Read the model definition and answer for the solid it produces. Units are mm, in the model's axes. Face numbers are marked on the shaded views. A direction names the side the tool comes from. Give positions to 0.01 mm unless a question says otherwise; leave off trailing zeros. Write each loop counter-clockwise with the first axis right and the second up, starting at its lowest first coordinate (ties: lowest second). Pieces come first, ordered by that corner, then holes. Notation, with made-up numbers: (48.25, -14) - (77.25, -14) arc R25 ccw to (77.25, 14) - close; hole circle Ø9 at (88.5, 84). An arc over 180 degrees is marked (long way). Answer as a JSON object with one key per item and string values. Group by question number.
```python
from build123d import *

# Parameters (mm, degrees)
F1_DEPTH     = 25
F2_R         = 5
F3_R         = 5
F4_R         = 2
F6_R         = 5
F7_DEPTH     = 20
F8_T1_DEPTH  = 16.879655815
F8_T3_DEPTH  = 23.3726224193
F8_T5_DEPTH  = 33.0268060681
F8_T10_DEPTH = 5.1
F8_T16_DEPTH = 5.1
F8_T22_DEPTH = 98.4210661838
F8_S23_R     = 20
F8_T24_DEPTH = 53
F8_S25_R     = 20
F8_T26_DEPTH = 53
F8_T30_DEPTH = 70.867251183
F8_S31_R     = 20
F8_T32_DEPTH = 39
F8_S33_R     = 20
F8_T34_DEPTH = 39


# Not quite as in the source:
# - a fillet or chamfer that OpenCascade refuses, or shapes differently, is made with other operations: its cross-section is extruded or revolved along the edge and cut away or added
# - two fillets or chamfers of one size are made in one step


with BuildPart() as f1:
    # F0 (on Top) → F1 (new body)
    with BuildSketch(Plane.XY):
        with BuildLine():
            ThreePointArc((-62.7989065684, 39.6886658546), (-81.243248627, 20.090620438), (-63.3367104763, 0))
            Line((-63.3367104763, 0), (0, -156.2183324342))
            Line((0, -156.2183324342), (63.3367104763, 0))
            ThreePointArc((63.3367104763, 0), (83.9060549488, 20.1553189736), (63.1791622356, 40.1485861756))
            ThreePointArc((63.1791622356, 40.1485861756), (68.8985621757, 62.3156526678), (50.0641206725, 75.3292680691))
            ThreePointArc((50.0641206725, 75.3292680691), (54.0847867027, 97.4676528526), (34.9687938538, 109.335788913))
            ThreePointArc((34.9687938538, 109.335788913), (37.8165399559, 130.8078112166), (19.4443891765, 142.2804515145))
            ThreePointArc((19.4443891765, 142.2804515145), (6.5496116272, 157.6455026462), (10.1508991793, 177.3784905672))
            ThreePointArc((10.1508991793, 177.3784905672), (-12.7726518652, 165.7418593556), (-21.8806297798, 141.7013702435))
            ThreePointArc((-21.8806297798, 141.7013702435), (-36.0248561638, 134.2091888045), (-40.144512278, 118.7424387834))
            Line((-40.144512278, 118.7424387834), (-34.6308081302, 107.732548238))
            ThreePointArc((-34.6308081302, 107.732548238), (-50.0933619749, 100.6048777691), (-54.4620472952, 84.1486070408))
            Line((-54.4620472952, 84.1486070408), (-50.2881059675, 75.0966394345))
            ThreePointArc((-50.2881059675, 75.0966394345), (-68.9068668709, 61.7610342158), (-62.7989065684, 39.6886658546))
        make_face()
        with BuildLine():
            Line((-19.4251702535, 141.7357782283), (-21.8806297798, 141.7013702435))
            ThreePointArc((-21.8806297798, 141.7013702435), (-20.6534286134, 141.7562965225), (-19.4251702535, 141.7357782283))
        make_face(mode=Mode.SUBTRACT)
        with BuildLine():
            ThreePointArc((-40.144512278, 118.7424387834), (-38.2560486822, 112.8026084286), (-34.6308081302, 107.732548238))
            Line((-34.6308081302, 107.732548238), (-40.144512278, 118.7424387834))
        make_face()
        with BuildLine():
            ThreePointArc((-54.4620472952, 84.1486070408), (-52.9480489841, 79.3584206811), (-50.2881059675, 75.0966394345))
            Line((-50.2881059675, 75.0966394345), (-54.4620472952, 84.1486070408))
        make_face()
        with BuildLine():
            ThreePointArc((-19.4251702535, 141.7357782283), (-20.6534286134, 141.7562965225), (-21.8806297798, 141.7013702435))
            Line((-21.8806297798, 141.7013702435), (-19.4251702535, 141.7357782283))
        make_face()
    extrude(amount=F1_DEPTH)

    # F2
    f2_edges = [f1.edges().sort_by_distance(p)[0] for p in [
        (10.150899, 177.378491, 12.5),
    ]]
    fillet(f2_edges, radius=F2_R)

    # F3
    f3_edges = [f1.edges().sort_by_distance(p)[0] for p in [
        (0, -156.218332, 12.5),
    ]]
    fillet(f3_edges, radius=F3_R)

    # F4
    f4_edges = [f1.edges().sort_by_distance(p)[0] for p in [
        (63.33671, 0, 12.5),
        (-63.33671, 0, 12.5),
    ]]
    fillet(f4_edges, radius=F4_R)

    # F6
    f6_edges = [f1.edges().sort_by_distance(p)[0] for p in [
        (19.444389, 142.280452, 12.5),
    ]]
    fillet(f6_edges, radius=F6_R)

    # F0 (on Top) → F7 (join)
    with BuildSketch(Plane.XY):
        with BuildLine():
            Line((-88.1787538528, 157.26955235), (-54.4620472952, 84.1486070408))
            ThreePointArc((-54.4620472952, 84.1486070408), (-50.0933619749, 100.6048777691), (-34.6308081302, 107.732548238))
            ThreePointArc((-34.6308081302, 107.732548238), (-38.2560486822, 112.8026084286), (-40.144512278, 118.7424387834))
            Line((-40.144512278, 118.7424387834), (-69.5091858506, 177.3784905672))
            Line((-69.5091858506, 177.3784905672), (-88.1787538528, 157.26955235))
        make_face()
    extrude(amount=F7_DEPTH)

    # F8: fillet of radius 5 on 5 edges, made by hand

    # F8_s2 → F8_t1 (cut)
    with BuildSketch(Plane(origin=(51.3609651153, 55.3207484048, 0), x_dir=(0, 0, 1), z_dir=(-0.6803920453, -0.7328483231, 0))):
        with BuildLine():
            ThreePointArc((20, 166.626604285), (18.5355339059, 170.1621381909), (15, 171.626604285))
            Line((15, 171.626604285), (20, 171.626604285))
            Line((20, 171.626604285), (20, 166.626604285))
        make_face()
    extrude(amount=F8_T1_DEPTH, mode=Mode.SUBTRACT)

    # F8_s4 → F8_t3 (cut)
    with BuildSketch(Plane.XY.offset(-8.3726224193)):
        with BuildLine():
            ThreePointArc((-85.9000875758, 159.72389727), (-87.1734696665, 157.1092566329), (-86.7763850028, 154.2282548314))
            Line((-86.7763850028, 154.2282548314), (-88.1787538528, 157.26955235))
            Line((-88.1787538528, 157.26955235), (-85.9000875758, 159.72389727))
        make_face()
    extrude(amount=F8_T3_DEPTH, mode=Mode.SUBTRACT)

    # F8_s6 → F8_t5 (cut)
    with BuildSketch(Plane.XY.offset(-18.0268060681)):
        with BuildLine():
            ThreePointArc((-66.280350029, 170.9310773526), (-70.0434123782, 173.6418343313), (-74.4153040312, 172.0941247282))
            Line((-74.4153040312, 172.0941247282), (-69.5091858506, 177.3784905672))
            Line((-69.5091858506, 177.3784905672), (-66.280350029, 170.9310773526))
        make_face()
    extrude(amount=F8_T5_DEPTH, mode=Mode.SUBTRACT)


with BuildPart() as f8_tool8:
    # F8_s9 → F8_t10 (new body)
    with BuildSketch(Plane.XY.offset(15)):
        Polygon((-82.2358459604, 156.3219370433), (-85.9733724081, 159.7919364745), (-88.2976120107, 157.2885046562), (-86.8671957836, 154.1863811872), align=None)
    extrude(amount=F8_T10_DEPTH)

    # F8_s11 → F8_t12 (revolve, cut)
    with BuildSketch(Plane(origin=(-82.2358459604, 156.3219370433, 15), x_dir=(0.9875247412, -0.1574639179, 0), z_dir=(-0.1574639179, -0.9875247412, 0))):
        with BuildLine():
            ThreePointArc((0, -5), (5, 0), (0, 5))
            Line((0, 5), (0, -5))
        make_face()
    revolve(axis=Axis((-82.2358459604, 156.3219370433, 15), (0, 0, 1)), mode=Mode.SUBTRACT)


with BuildPart() as f1_1:
    add(f1.part)

    # F8_t7: cut F8_tool8
    add(f8_tool8.part, mode=Mode.SUBTRACT)


with BuildPart() as f8_tool14:
    # F8_s15 → F8_t16 (new body)
    with BuildSketch(Plane.XY.offset(15)):
        Polygon((-70.7510624158, 168.6921645015), (-74.4885888636, 172.1621639327), (-69.4843483193, 177.5522170885), (-66.1909357813, 170.9758556096), align=None)
    extrude(amount=F8_T16_DEPTH)

    # F8_s17 → F8_t18 (revolve, cut)
    with BuildSketch(Plane(origin=(-70.7510624158, 168.6921645015, 15), x_dir=(-0.1415300075, -0.989933966, 0), z_dir=(-0.989933966, 0.1415300075, 0))):
        with BuildLine():
            ThreePointArc((0, -5), (5, 0), (0, 5))
            Line((0, 5), (0, -5))
        make_face()
    revolve(axis=Axis((-70.7510624158, 168.6921645015, 15), (0, 0, 1)), mode=Mode.SUBTRACT)


with BuildPart() as f1_2:
    add(f1_1.part)

    # F8_t13: cut F8_tool14
    add(f8_tool14.part, mode=Mode.SUBTRACT)


with BuildPart() as f8_tool20:
    # F8_s21 → F8_t22 (new body)
    with BuildSketch(Plane(origin=(-73.8618913818, 160.1832406418, 0), x_dir=(0, 0, 1), z_dir=(0.4187364424, -0.9081078085, 0))):
        with BuildLine():
            ThreePointArc((20, 9.2213220725), (18.5355339059, 12.7568559784), (15, 14.2213220725))
            Line((15, 14.2213220725), (20, 14.2213220725))
            Line((20, 14.2213220725), (20, 9.2213220725))
        make_face()
    extrude(amount=F8_T22_DEPTH)

    # F8_s23 → F8_t24 (cut, symmetric)
    with BuildSketch(Plane.XY.offset(17.5)):
        with Locations((-34.7858928144, 87.7331495285)):
            Circle(F8_S23_R)
    extrude(amount=F8_T24_DEPTH, both=True, mode=Mode.SUBTRACT)

    # F8_s25 → F8_t26 (cut, symmetric)
    with BuildSketch(Plane.XY.offset(17.5)):
        with Locations((-50.049379468, 55.0980642438)):
            Circle(F8_S25_R)
    extrude(amount=F8_T26_DEPTH, both=True, mode=Mode.SUBTRACT)


with BuildPart() as f1_3:
    add(f1_2.part)

    # F8_t19: cut F8_tool20
    add(f8_tool20.part, mode=Mode.SUBTRACT)


with BuildPart() as f8_tool28:
    # F8_s29 → F8_t30 (new body)
    with BuildSketch(Plane(origin=(-49.9943289817, 99.8298195219, 0), x_dir=(0, 0, 1), z_dir=(-0.4477825702, 0.8941424774, 0))):
        with BuildLine():
            ThreePointArc((15, 17.2758807713), (18.5355339059, 15.8114146772), (20, 12.2758807713))
            Line((20, 12.2758807713), (20, 17.2758807713))
            Line((20, 17.2758807713), (15, 17.2758807713))
        make_face()
    extrude(amount=F8_T30_DEPTH)

    # F8_s31 → F8_t32 (cut, symmetric)
    with BuildSketch(Plane.XY.offset(17.5)):
        with Locations((-20.3731991351, 121.7582598329)):
            Circle(F8_S31_R)
    extrude(amount=F8_T32_DEPTH, both=True, mode=Mode.SUBTRACT)

    # F8_s33 → F8_t34 (cut, symmetric)
    with BuildSketch(Plane.XY.offset(17.5)):
        with Locations((-34.7858928144, 87.7331495285)):
            Circle(F8_S33_R)
    extrude(amount=F8_T34_DEPTH, both=True, mode=Mode.SUBTRACT)


with BuildPart() as f1_4:
    add(f1_3.part)

    # F8_t27: cut F8_tool28
    add(f8_tool28.part, mode=Mode.SUBTRACT)


solid = f1_4.part
```
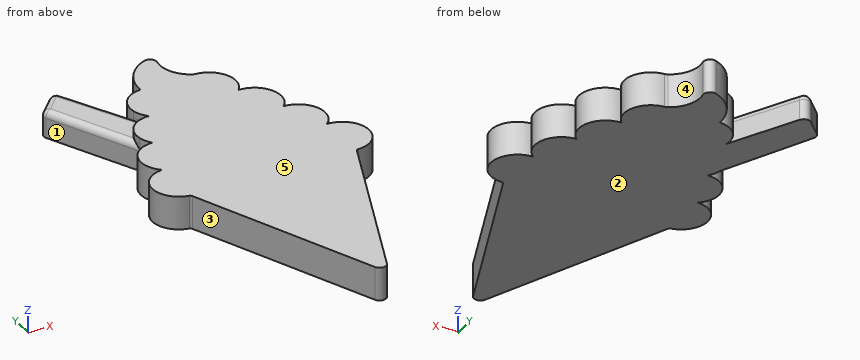
1) For a pull along Y with two mould halves and no side action, classify the marked faces 3, 4 and 5 as released by +Y, released by -Y, zero draft, split by the parting line, or undercut.
2) Find the intervals of material crossed by line 1 (X direction, y = 160, z = 11); line 2 (X direction, y = 146, z = 1.75); line 3 (X direction, y = 70.5, z = 10), in increasing order. Write a range as [from, to].
3) Flat-ended cylindrical pins translate along their axes: pin 1 Ø12 at (y, z) = (-57.5, 2.5) entering from -X; pin 2 Ø2 at (x, z) = (44.5, 12) entering from -Y; pin 3 Ø1.5 at (x, z) = (22.5, 4) entering from +Y. Find the tip coordinate at first contact, or state that the pin passes through.
4) Find section B-B, the plane y = 58. Write down the section's boundary in (x, z), and give its area (3 significant figures).
5) Find section A-A, the plane x = -12.5. Write down the section's boundary in (y, z).
6) Which of the six approach directions +Z, -Z, +X, -X, +Y, -Y give full straight-line access (tool end or side, diameter ignored) to the marked faces 1 and 2?
Values follow:
{
 "1": {"face 3": "released by -Y", "face 4": "undercut", "face 5": "zero draft"},
 "2": {"line 1": "x = [-85.64, -60.81], [-16.97, 6.05]", "line 2": "x = [-82.98, -53.79], [-21.65, 13.74]", "line 3": "x = [-62.81, 63.19]"},
 "3": {"pin 1": "stops at x = -42.46", "pin 2": "stops at y = -48.93", "pin 3": "stops at y = 142.18"},
 "4": {"outline": "(-69.84, 0) - (69.98, 0) - (69.98, 25) - (-69.84, 25) - close", "area": "3,500 mm2"},
 "5": {"outline": "(-125.39, 0) - (166.04, 0) - (166.04, 25) - (-125.39, 25) - close"},
 "6": {"face 1": "+Z, -Z, -X", "face 2": "-Z, +X, -X, +Y, -Y"}
}
